Check sheet for the modelled part. Datum: model origin and axes. Units: mm. A direction names the side the tool comes from. Round coordinates to 2 decimals unless told otherwise and drop trailing zeros. Loops run counter-clockwise (first coordinate to the right, second up) from the corner with the lowest first, then second, coordinate; pieces in that order, holes last. Notation, with made-up numbers: (39.5, 64) -> (43.5, 64) arc R30 cw to (43.5, 94) -> close; hole circle Ø9 at (65, 3.5). An arc over 180 degrees is marked (long way). Return JSON: item names as keys, results as strings.
from build123d import *

# Parameters (mm, degrees)
F1_DEPTH = 5.715
F3_DEPTH = 5.3975
F4_W     = 5.08
F4_H     = 137.2235
F5_DEPTH = 63.165533


with BuildPart() as f1:
    # F0 (on Front) → F1 (new body)
    with BuildSketch(Plane.XZ):
        Polygon((30.312766, 68.7705), (-33.170266, 68.7705), (-33.170266, -68.7705), (-30.630266, -68.7705), (-30.630266, -63.478089), (30.312766, 63.50442), align=None)
    extrude(amount=F1_DEPTH)

    # F2 (on face) → F3 (cut)
    with BuildSketch(Plane.XZ.offset(5.715)):
        Polygon((24.928634, 52.2859), (-29.177386, 52.2859), (-29.177386, -60.45083), align=None)
    extrude(amount=-F3_DEPTH, mode=Mode.SUBTRACT)

    # F4 (on face) → F5 (cut)
    with BuildSketch(Plane.YZ.offset(30.312766)):
        with Locations((-2.8575, -0.15875)):
            Rectangle(F4_W, F4_H)
    extrude(amount=-F5_DEPTH, mode=Mode.SUBTRACT)


solid = f1.part
Q1. Material ranges on line 1 (Y direction, x = -25, z = 57) (1 decimal); line 2 (X direction, y = -4.75, z = -16); line 3 (Z direction, x = -18.5, y = -3.4), recorded low to high.
Results list:
{"line 1": "-5.7 to -5.4, -0.3 to 0", "line 2": "-33.17 to -32.85", "line 3": "68.45 to 68.77"}
Q2. Tool access check on faces 5 (the flat face through (27.583, -5.554, 57.817)), 6 (the flat face through (-32, -5.398, 35)). Record the directions out of +Z, -Z, +X, -X, +Y, -Y that give a thin tool (end or side, any length) a straight path to the whole face; none if there is none.
Results list:
{"face 5": "-Z, +X, +Y, -Y", "face 6": "-Z, +X"}
Q3. Section check C-C (y = -3.85). Record the boundary of the cut face in (x, z).
Results list:
{"outline": "(-33.17, -68.77) -> (-32.85, -68.77) -> (-32.85, 68.45) -> (30.31, 68.45) -> (30.31, 68.77) -> (-33.17, 68.77) -> close"}
Q4. Go/stop test with a flat-tipped pin: pin 1 (1.5 mm diameter, centred on x = -5.5, y = -3.5, fed in from -Z). Record where the tip stops, or that it passes through.
Results list:
{"pin 1": "z = 68.45"}
Q5. Draft check along Y on faces 1 (the flat face through (-9, 0, 16)), 2 (the flat face through (-8, -0.317, 29)), 3 (the flat face through (-32.853, -3, 1)), 4 (the flat face through (-0.585, -0.157, -0.876)). Enter one of: released by +Y, released by -Y, zero draft, split by the parting line, or undercut.
Results list:
{"face 1": "released by +Y", "face 2": "undercut", "face 3": "undercut", "face 4": "zero draft"}
